Autodesk Inventor part; units mm, degrees
ref_plane "YZ Plane" through (0, 0, 0) normal (1, 0, 0) x (0, 1, 0)
ref_plane "XZ Plane" through (0, 0, 0) normal (0, 1, 0) x (-1, 0, 0)
ref_plane "XY Plane" through (0, 0, 0) normal (0, 0, 1) x (1, 0, 0)
sketch "Sketch1" plane through (0, 0, 0) normal (0, 1, 0) x (-1, 0, 0)
  circle A0 centre (0, 0) radius 7
  dimension "d0" = 14
extrude "Extrusion1" add sketch "Sketch1" along normal blind 8.5
sketch "Sketch2" plane through (0, 8.5, 0) normal (0, 1, 0) x (1, 0, 0)
  circle A0 centre (0, 0) radius 4
  dimension "d3" = 8
extrude "Extrusion2" cut sketch "Sketch2" against normal blind 3
sketch "Sketch3" plane through (0, 5.5, 0) normal (0, 1, 0) x (1, 0, 0)
  circle A0 centre (0, 0) radius 2
  dimension "d6" = 4
extrude "Extrusion3" cut sketch "Sketch3" against normal through all
sketch "Sketch4" plane through (0, 0, 0) normal (0, -1, 0) x (1, 0, 0)
  circle A0 centre (0, 0) radius 2
  circle A1 centre (0, 0) radius 10
  circle A2 centre (0, 0) radius 7
  dimension "d9" = 20
extrude "Extrusion4" add sketch "Sketch4" against normal blind 2 contours A1
chamfer "Chamfer1" distance 2 angle 45 1 edges at (-10, 2, 0)
properties part number "spacer_long"
Input: part model. Units: mm. Frame: model coordinates. A direction names the side the tool comes from. Give positions to 0.01 mm unless a question says otherwise; leave off trailing zeros. Order: outer loops, then holes, each group sorted by start corner. A loop starts at its lowest first (then second) coordinate and runs counter-clockwise, first axis right, second up.
Q1. Section C-C on y = 3.5. Output: boundary loops of the cut face in (x, z), and give its area (3 significant figures).
Checked values:
outline: circle Ø14 at (0, 0); hole circle Ø4 at (0, 0)
area: 141 mm2
Q2. Ray query, probe 1 along Z at (x, y) = (0, 2.95); probe 2 along Z at (x, y) = (0, 7.9). Return the intervals inside material, ascending.
Checked values:
probe 1: z = -7 to -2, 2 to 7
probe 2: z = -7 to -4, 4 to 7
Q3. Section D-D on y = 1.5. Output: boundary loops of the cut face in (x, z).
Checked values:
outline: circle Ø17 at (0, 0); hole circle Ø4 at (0, 0)
Q4. Set-up query: faces 4 (the flat face through (-0.1, 0, 2.4)), 5 (the cylindrical face through (-0.867, 7.021, 3.905)). Return all of +Z, -Z, +X, -X, +Y, -Y with unobstructed straight access to the full face (end or side cutting, diameter ignored); none if empty.
Checked values:
face 4: +Z, -Z, +X, -X, -Y
face 5: +Y
Q5. Contact query for flat-ended pins moving along their axis: pin 1 Ø6 at (x, z) = (2, -1) entering from +Y; pin 2 Ø1.5 at (y, z) = (2, 1.5) entering from +X. Output: stop coordinate, or through.
Checked values:
pin 1: stops at y = 8.5
pin 2: stops at x = 8.63
Q6. Draft query along Z for faces 1 (the flat face through (-2, 5.5, 1)), 2 (the cylindrical face through (-6.466, 5.204, 2.681)), 3 (the flat face through (-3, 8.5, -3)). Return one class per face: +Z half, -Z half, draft (parallel to the pull), parting line (faces both ways), or undercut.
Checked values:
face 1: undercut
face 2: parting line
face 3: draft
